Geometry: final body of the model. Coordinates: model frame, mm. Give positions to 0.01 mm unless a question says otherwise; leave off trailing zeros. Loops run counter-clockwise (first coordinate to the right, second up) from the corner with the lowest first, then second, coordinate; pieces in that order, holes last.
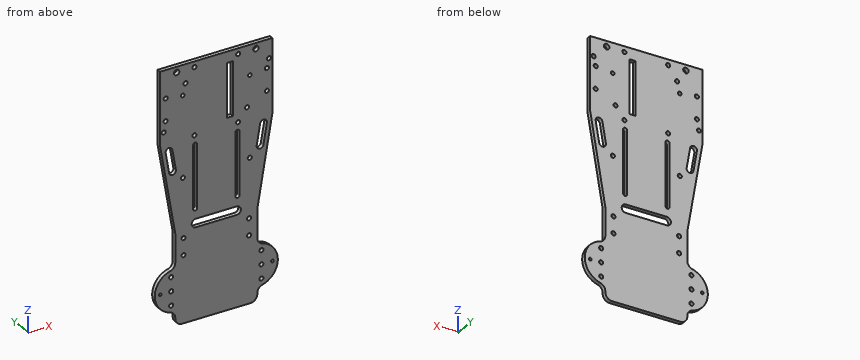
from build123d import *

# Parameters (mm, degrees)
BOSS_EXTRUDE1_DEPTH  = 3
BOSS_EXTRUDE2_DEPTH  = 60
BOSS_EXTRUDE3_DEPTH  = 3
SKETCH4_R            = 1.5
CUT_EXTRUDE1_DEPTH   = 4
LPATTERN1_COUNT      = 2
LPATTERN1_PITCH      = 48
LPATTERN1_COUNT_DIR2 = 2
LPATTERN1_PITCH_DIR2 = 12
SKETCH6_W            = 23.651553975
SKETCH6_H            = 52.455294706
CUT_EXTRUDE2_DEPTH   = 4
SKETCH8_W            = 46.628396315
SKETCH8_H            = 3
BOSS_EXTRUDE4_DEPTH  = 19
SKETCH9_W            = 8
SKETCH9_H            = 3
BOSS_EXTRUDE5_DEPTH  = 4.651554
SKETCH12_R           = 1.5
CUT_EXTRUDE4_DEPTH   = 17
SKETCH13_R           = 1
SKETCH13_R_2         = 1.5
CUT_EXTRUDE5_DEPTH   = 4
SKETCH14_R           = 1.35
CUT_EXTRUDE6_DEPTH   = 17
SKETCH15_R           = 1.5
CUT_EXTRUDE7_DEPTH   = 17
SKETCH16_R           = 1.5
CUT_EXTRUDE8_DEPTH   = 17
CUT_EXTRUDE9_DEPTH   = 17
SKETCH19_R           = 1.5
CUT_EXTRUDE10_DEPTH  = 17
CUT_EXTRUDE11_START  = -65.281828
SKETCH20_W           = 42
SKETCH20_H           = 16
CUT_EXTRUDE11_DEPTH  = 70.563656
FILLET1_R            = 5
FILLET2_R            = 5
SKETCH21_R           = 1.5
CUT_EXTRUDE12_DEPTH  = 4
CUT_EXTRUDE13_DEPTH  = 4
SKETCH23_R           = 1.5
CUT_EXTRUDE14_DEPTH  = 4
CUT_EXTRUDE15_DEPTH  = 4
SKETCH25_R           = 2
CUT_EXTRUDE16_DEPTH  = 4


with BuildPart() as part:
    # Sketch1 → Boss-Extrude1 (new body)
    with BuildSketch(Plane(origin=(0, 0, 0), x_dir=(1, 0, 0), z_dir=(0, 1, 0))):
        with BuildLine():
            Line((-41, 0), (41, 0))
            Line((41, 0), (41, 53))
            Line((41, 53), (30, 117.062469512))
            Line((30, 117.062469512), (30, 137.635083269))
            ThreePointArc((30, 137.635083269), (31.047152925, 140.696945447), (33.75, 142.476312452))
            ThreePointArc((33.75, 142.476312452), (45, 157), (33.75, 171.523687548))
            ThreePointArc((33.75, 171.523687548), (31.047152925, 173.303054553), (30, 176.364916731))
            Line((30, 176.364916731), (30, 182))
            Line((30, 182), (-30, 182))
            Line((-30, 182), (-30, 176.364916731))
            ThreePointArc((-30, 176.364916731), (-31.047152925, 173.303054553), (-33.75, 171.523687548))
            ThreePointArc((-33.75, 171.523687548), (-45, 157), (-33.75, 142.476312452))
            ThreePointArc((-33.75, 142.476312452), (-31.047152925, 140.696945447), (-30, 137.635083269))
            Line((-30, 137.635083269), (-30, 117.062469512))
            Line((-30, 117.062469512), (-41, 53))
            Line((-41, 53), (-41, 0))
        make_face()
    extrude(amount=BOSS_EXTRUDE1_DEPTH)

    # Sketch4 → Cut-Extrude1 (cut, through all)
    with BuildSketch(Plane(origin=(0, 3, 0), x_dir=(1, 0, 0), z_dir=(0, 1, 0))):
        with Locations((-24, 134)):
            Circle(SKETCH4_R)
    cut_extrude1 = extrude(amount=-CUT_EXTRUDE1_DEPTH, mode=Mode.SUBTRACT)

    # LPattern1: Cut-Extrude1 2 × 2
    with Locations(*[(i * LPATTERN1_PITCH, 0, j * LPATTERN1_PITCH_DIR2) for i in range(LPATTERN1_COUNT) for j in range(LPATTERN1_COUNT_DIR2) if (i, j) != (0, 0)]):
        add(cut_extrude1, mode=Mode.SUBTRACT)

    # Sketch6 → Cut-Extrude2 (cut, through all)
    with BuildSketch(Plane(origin=(0, 3, 0), x_dir=(1, 0, 0), z_dir=(0, 1, 0))):
        with Locations((0.55948687, 20.400748962)):
            Rectangle(SKETCH6_W, SKETCH6_H)
    extrude(amount=-CUT_EXTRUDE2_DEPTH, mode=Mode.SUBTRACT)

    # Sketch8 → Boss-Extrude4 (add)
    with BuildSketch(Plane(origin=(-11.266290117, 0, 0), x_dir=(0, 0, -1), z_dir=(1, 0, 0))):
        with Locations((23.314198158, 1.5)):
            Rectangle(SKETCH8_W, SKETCH8_H)
    extrude(amount=BOSS_EXTRUDE4_DEPTH)

    # Sketch9 → Boss-Extrude5 (add)
    with BuildSketch(Plane(origin=(7.733709883, 0, 0), x_dir=(0, 0, -1), z_dir=(1, 0, 0))):
        with Locations((4, 1.5)):
            Rectangle(SKETCH9_W, SKETCH9_H)
    extrude(amount=BOSS_EXTRUDE5_DEPTH)

    # Sketch12 → Cut-Extrude4 (cut, through all)
    with BuildSketch(Plane.XZ):
        with Locations((-16, -4)):
            Circle(SKETCH12_R)
        with Locations((16, -4)):
            Circle(SKETCH12_R)
    extrude(amount=-CUT_EXTRUDE4_DEPTH, mode=Mode.SUBTRACT)

    # Sketch13 → Cut-Extrude5 (cut, through all)
    with BuildSketch(Plane(origin=(0, 3, 0), x_dir=(1, 0, 0), z_dir=(0, 1, 0))):
        with Locations((41, 157)):
            Circle(SKETCH13_R)
        with Locations((-41, 157)):
            Circle(SKETCH13_R)
        with Locations((33, 157)):
            Circle(SKETCH13_R_2)
        with Locations((-33, 156.913211427)):
            Circle(SKETCH13_R_2)
        with Locations((33, 147)):
            Circle(SKETCH13_R_2)
        with Locations((33, 167)):
            Circle(SKETCH13_R_2)
        with Locations((-33, 166.913211427)):
            Circle(SKETCH13_R_2)
        with Locations((-33, 146.913211427)):
            Circle(SKETCH13_R_2)
    extrude(amount=-CUT_EXTRUDE5_DEPTH, mode=Mode.SUBTRACT)

    # Sketch14 → Cut-Extrude6 (cut, through all)
    with BuildSketch(Plane.XZ):
        with Locations((-24.5, -21.5)):
            Circle(SKETCH14_R)
        with Locations((24.54, -21.4)):
            Circle(SKETCH14_R)
    extrude(amount=-CUT_EXTRUDE6_DEPTH, mode=Mode.SUBTRACT)

    # Sketch15 → Cut-Extrude7 (cut, through all)
    with BuildSketch(Plane.XZ):
        with Locations((22.5, -43.5)):
            Circle(SKETCH15_R)
        with Locations((38.5, -13.5)):
            Circle(SKETCH15_R)
    extrude(amount=-CUT_EXTRUDE7_DEPTH, mode=Mode.SUBTRACT)

    # Sketch16 → Cut-Extrude8 (cut, through all)
    with BuildSketch(Plane.XZ):
        with Locations((-22.5, -13.5)):
            Circle(SKETCH16_R)
        with Locations((-38.5, -43.5)):
            Circle(SKETCH16_R)
    extrude(amount=-CUT_EXTRUDE8_DEPTH, mode=Mode.SUBTRACT)

    # Sketch17 → Cut-Extrude9 (cut, through all)
    with BuildSketch(Plane.XZ):
        with BuildLine():
            Line((37.02491368, -58.423076923), (34.486452142, -73.206723734))
            ThreePointArc((34.486452142, -73.206723734), (31.599434084, -75.247587946), (29.558569872, -72.360569887))
            Line((29.558569872, -72.360569887), (32.09703141, -57.576923077))
            ThreePointArc((32.09703141, -57.576923077), (34.984049468, -55.536058865), (37.02491368, -58.423076923))
        make_face()
        with BuildLine():
            Line((-37.02491368, -58.423076923), (-34.486452142, -73.206723734))
            ThreePointArc((-34.486452142, -73.206723734), (-31.599434084, -75.247587946), (-29.558569872, -72.360569887))
            Line((-29.558569872, -72.360569887), (-32.09703141, -57.576923077))
            ThreePointArc((-32.09703141, -57.576923077), (-34.984049468, -55.536058865), (-37.02491368, -58.423076923))
        make_face()
    extrude(amount=-CUT_EXTRUDE9_DEPTH, mode=Mode.SUBTRACT)

    # Sketch19 → Cut-Extrude10 (cut, through all)
    with BuildSketch(Plane(origin=(0, 0, 0), x_dir=(-1, 0, 0), z_dir=(0, -1, 0))):
        with Locations((24.5, 79.5)):
            Circle(SKETCH19_R)
        with Locations((-24.5, 79.5)):
            Circle(SKETCH19_R)
    extrude(amount=-CUT_EXTRUDE10_DEPTH, mode=Mode.SUBTRACT)

    # Fillet1
    fillet1_edges = [part.edges().sort_by_distance(p)[0] for p in [
        (30, 1.5, -182),
    ]]
    fillet(fillet1_edges, radius=FILLET1_R)

    # Fillet2
    fillet2_edges = [part.edges().sort_by_distance(p)[0] for p in [
        (-30, 1.5, -182),
    ]]
    fillet(fillet2_edges, radius=FILLET2_R)

    # Sketch21 → Cut-Extrude12 (cut, through all)
    with BuildSketch(Plane(origin=(0, 3, 0), x_dir=(1, 0, 0), z_dir=(0, 1, 0))):
        with Locations((37, 20)):
            Circle(SKETCH21_R)
        with Locations((-37, 20)):
            Circle(SKETCH21_R)
        with Locations((-37, 36)):
            Circle(SKETCH21_R)
        with Locations((37, 36)):
            Circle(SKETCH21_R)
    extrude(amount=-CUT_EXTRUDE12_DEPTH, mode=Mode.SUBTRACT)

    # Sketch22 → Cut-Extrude13 (cut, through all)
    with BuildSketch(Plane(origin=(0, 3, 0), x_dir=(1, 0, 0), z_dir=(0, 1, 0))):
        with BuildLine():
            Line((14, 58.7), (14, 103.7))
            ThreePointArc((14, 103.7), (15.5, 105.2), (17, 103.7))
            Line((17, 103.7), (17, 58.7))
            ThreePointArc((17, 58.7), (15.5, 57.2), (14, 58.7))
        make_face()
        with BuildLine():
            Line((-17, 58.7), (-17, 103.7))
            ThreePointArc((-17, 103.7), (-15.5, 105.2), (-14, 103.7))
            Line((-14, 103.7), (-14, 58.7))
            ThreePointArc((-14, 58.7), (-15.5, 57.2), (-17, 58.7))
        make_face()
    extrude(amount=-CUT_EXTRUDE13_DEPTH, mode=Mode.SUBTRACT)

    # Sketch23 → Cut-Extrude14 (cut, through all)
    with BuildSketch(Plane(origin=(0, 3, 0), x_dir=(1, 0, 0), z_dir=(0, 1, 0))):
        with Locations((-16, 52)):
            Circle(SKETCH23_R)
        with Locations((16, 52)):
            Circle(SKETCH23_R)
    extrude(amount=-CUT_EXTRUDE14_DEPTH, mode=Mode.SUBTRACT)

    # Sketch24 → Cut-Extrude15 (cut, through all)
    with BuildSketch(Plane(origin=(0, 3, 0), x_dir=(1, 0, 0), z_dir=(0, 1, 0))):
        with BuildLine():
            Line((15, 111), (-15, 111))
            ThreePointArc((-15, 111), (-18, 114), (-15, 117))
            Line((-15, 117), (15, 117))
            ThreePointArc((15, 117), (18, 114), (15, 111))
        make_face()
    extrude(amount=-CUT_EXTRUDE15_DEPTH, mode=Mode.SUBTRACT)

    # Sketch25 → Cut-Extrude16 (cut, through all)
    with BuildSketch(Plane(origin=(0, 3, 0), x_dir=(1, 0, 0), z_dir=(0, 1, 0))):
        with Locations((-29, 4)):
            Circle(SKETCH25_R)
        with Locations((29, 4)):
            Circle(SKETCH25_R)
    extrude(amount=-CUT_EXTRUDE16_DEPTH, mode=Mode.SUBTRACT)


with BuildPart() as body_2:
    # Sketch2 → Boss-Extrude2 (new body)
    with BuildSketch(Plane.ZY.offset(30)):
        Polygon((-182, 0), (-196, 13), (-196, 16), (-182, 3), align=None)
    extrude(amount=-BOSS_EXTRUDE2_DEPTH)

    # Sketch3 → Boss-Extrude3 (add)
    with BuildSketch(Plane(origin=(0, 16, 0), x_dir=(1, 0, 0), z_dir=(0, 1, 0))):
        with BuildLine():
            Line((-30, 196), (30, 196))
            Line((30, 196), (34.802113349, 210.939908196))
            ThreePointArc((34.802113349, 210.939908196), (33.362697678, 219.890631628), (25.281827736, 224))
            Line((25.281827736, 224), (-25.281827736, 224))
            ThreePointArc((-25.281827736, 224), (-33.362697678, 219.890631628), (-34.802113349, 210.939908196))
            Line((-34.802113349, 210.939908196), (-30, 196))
        make_face()
    extrude(amount=-BOSS_EXTRUDE3_DEPTH)

    # Sketch20 → Cut-Extrude11 (cut)
    with BuildSketch(Plane(origin=(30, 0, 0), x_dir=(0, 0, -1), z_dir=(1, 0, 0)).offset(CUT_EXTRUDE11_START)):
        with Locations((203, 8)):
            Rectangle(SKETCH20_W, SKETCH20_H)
    extrude(amount=CUT_EXTRUDE11_DEPTH, mode=Mode.SUBTRACT)


solid = part.part
Item 1: Ray query, probe 1 along X at (y, z) = (2.3, -36); probe 2 along X at (y, z) = (2.55, -31.5); probe 3 along Z at (x, y) = (12, 0.5). Return the intervals inside material, ascending.
Values follow:
probe 1: x = -41 to -38.5, -35.5 to 7.73, 12.39 to 35.5, 38.5 to 41
probe 2: x = -41 to 7.73, 12.39 to 41
probe 3: z = -182 to -117, -111 to -46.63, -8 to 0
Item 2: Pin query (flat end, axial travel): pin 1 (1.8 mm diameter, centred on x = 33, z = -147, fed in from -Y); pin 2 (0.9 mm diameter, centred on y = 1.5, z = -21, fed in from -X). Return the tip coordinate at first contact, or that it passes through.
Values follow:
pin 1: passes through
pin 2: stops at x = -41
Item 3: Section query C-C on y = 1.7. Give the number of separate pieces and of enclosed holes in the cut face, plus the area to 3 significant figures.
Values follow:
separate pieces: 1
enclosed holes: 36
area: 12,400 mm2
Item 4: Section query A-A on x = 0.5. Return loops of the section in (y, z).
Values follow:
outline: (0, -182) - (3, -182) - (3, -117) - (0, -117) - close; (0, -111) - (3, -111) - (3, 0) - (0, 0) - close
Item 5: Section query B-B on z = -127.5. Return loops of the section in (x, y), plus the area to 3 significant figures.
Values follow:
outline: (-30, 0) - (30, 0) - (30, 3) - (-30, 3) - close
area: 180 mm2
